```python
from build123d import *

# Parameters (mm, degrees)
SKETCH_1_W          = 75
SKETCH_1_H          = 75
EXTRUDE_1_DEPTH     = 10
SKETCH_2_R          = 1.6
CUT_EXTRUDE_1_DEPTH = 10
SKETCH_3_W          = 12.7
SKETCH_3_H          = 12.7
EXTRUDE_2_DEPTH     = 20


with BuildPart() as part:
    # Эскиз1 → Бобышка-Вытянуть1 (new body)
    with BuildSketch(Plane(origin=(0, 0, 0), x_dir=(1, 0, 0), z_dir=(0, 1, 0))):
        with Locations((2.261306533, -8.291457286)):
            Rectangle(SKETCH_1_W, SKETCH_1_H)
    extrude(amount=EXTRUDE_1_DEPTH)

    # Эскиз2 → Вырез-Вытянуть1 (cut)
    with BuildSketch(Plane(origin=(0, 10, 0), x_dir=(1, 0, 0), z_dir=(0, 1, 0))):
        with Locations(Location((-25.238693467, 19.208542714, 0), (0, 0, 270))):
            Circle(SKETCH_2_R)
        with Locations(Location((29.761306533, 19.208542714, 0), (0, 0, 270))):
            Circle(SKETCH_2_R)
        with Locations(Location((-25.238693467, -35.791457286, 0), (0, 0, 270))):
            Circle(SKETCH_2_R)
        with Locations(Location((29.761306533, -35.791457286, 0), (0, 0, 270))):
            Circle(SKETCH_2_R)
    extrude(amount=-CUT_EXTRUDE_1_DEPTH, mode=Mode.SUBTRACT)

    # Эскиз3 → Бобышка-Вытянуть2 (add)
    with BuildSketch(Plane(origin=(0, 10, 0), x_dir=(1, 0, 0), z_dir=(0, 1, 0))):
        with Locations((2.261306533, -8.291457286)):
            Rectangle(SKETCH_3_W, SKETCH_3_H)
    extrude(amount=EXTRUDE_2_DEPTH)


solid = part.part
```
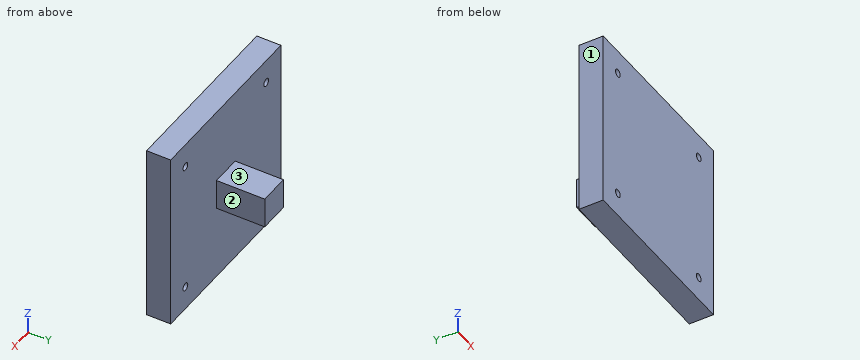
Geometry check sheet. Reference: the model listing, model coordinates, mm. Face numbers are marked on the shaded views. A direction names the side the tool comes from. Give positions to 0.01 mm unless a question says otherwise; leave off trailing zeros. Loops run counter-clockwise (first coordinate to the right, second up) from the corner with the lowest first, then second, coordinate; pieces in that order, holes last. Notation, with made-up numbers: M 76.5,84.5 L 111.5,84.5 A30 ccw 111.5,118.5 Z; hole C 65,28 d5. An arc over 180 degrees is marked long. Answer as CSV lines item,"result".
Item 1: Material ranges on line 1 (Y direction, x = 25.5, z = 11); line 2 (Z direction, x = 4.5, y = 17.5); line 3 (X direction, y = 17.5, z = 8), recorded low to high.
Values:
line 1,"y = 0 to 10"
line 2,"z = 1.94 to 14.64"
line 3,"x = -4.09 to 8.61"
Item 2: Depth check by flat-ended pin: P1, Ø4, axis at y = 21.5, z = 7, coming from the +X side; P2, Ø3.5, axis at x = -25.24, z = 35.79, coming from the +Y side; P3, Ø4, axis at x = 29.76, z = 35.79, coming from the -Y side; P4, Ø6.5, axis at x = 1.5, y = 24.5, coming from the -Z side. Enter the tip coordinate at first touch or a pass-through.
Values:
P1,"stops at x = 8.61"
P2,"stops at y = 10"
P3,"stops at y = 0"
P4,"stops at z = 1.94"
Item 3: Access from +Z, -Z, +X, -X, +Y, -Y to the whole of each face (thin tool, end or side, straight path). Record for the marked faces 1, 2 and 3.
Values:
face 1,"+Z, -Z, -X, +Y, -Y"
face 2,"+Z, -Z, +X, +Y"
face 3,"+Z, +X, -X, +Y"
Item 4: Cross-section at A-A on z = 12. Record the cut outline in (x, y), and give its area (3 significant figures).
Values:
outline,"M -35.24,0 L 39.76,0 L 39.76,10 L 8.61,10 L 8.61,30 L -4.09,30 L -4.09,10 L -35.24,10 Z"
area,"1,000 mm²"
Item 5: Cross-section at C-C on y = 22. Record the cut outline in (x, z).
Values:
outline,"M -4.09,1.94 L 8.61,1.94 L 8.61,14.64 L -4.09,14.64 Z"
Item 6: Cross-section at B-B on x = 21. Record the cut outline in (y, z).
Values:
outline,"M 0,-29.21 L 10,-29.21 L 10,45.79 L 0,45.79 Z"
